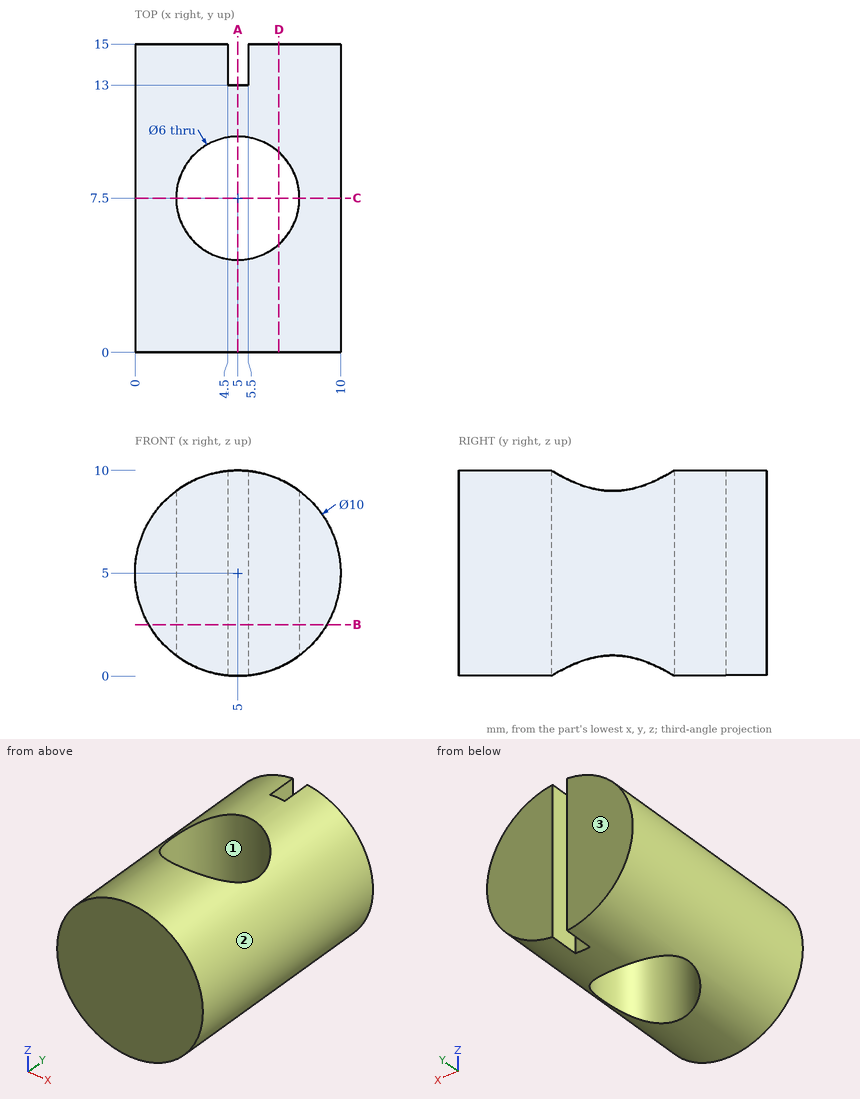
Could you check a few things on this drawing? It's one solid part, dimensions in mm from its lowest x, y, z. Coordinates: 2 decimals unless noted, no trailing zeros. Write each loop counter-clockwise with the first axis right and the second up, starting at its lowest first coordinate (ties: lowest second). Pieces come first, ordered by that corner, then holes. Notation, with made-up numbers: (2, 46) - (15, 46) arc R35 cw to (15, 78) - close; hole circle Ø11 at (87.5, 45). An arc over 180 degrees is marked (long way). Return JSON: item names as keys, results as strings. Group by question number.
Item 1: If we section it at A-A (x = 5): Write out the boundary of the cut face in (y, z).
Item 2: If we section it at B-B (z = 2.5): Write out the boundary of the cut face in (x, y), then the cut area to 3 significant figures.
Item 3: If we section it at C-C (y = 7.5): Write out the boundary of the cut face in (x, z).
Item 4: We'd pull the mould along X, two halves only. Please class the marked faces 1, 2 and 3: pulls with the +X half, pulls with the -X half, needs draft (parallel to the pull), parting line crosses it, or undercut.
Item 5: Please list where these lines run through material, in increasing order: probe 1 along Y at (x, z) = (5, 6.5); probe 2 along Y at (x, z) = (7, 4); probe 3 along Z at (x, y) = (1, 5.5).
Item 6: I'm going to push flat-ended pins straight in: pin 1 Ø3 at (y, z) = (3.5, 1.5) entering from -X; pin 2 Ø3 at (y, z) = (6, 8) entering from -X; pin 3 Ø0.5 at (x, z) = (5, 6.5) entering from +Y. Where does each tip first touch, or does it pass through?
Item 7: If we section it at D-D (x = 7): Write out the boundary of the cut face in (y, z), then the cut area to 3 significant figures.
Return value:
{
 "1": {"outline": "(0, 0) - (4.5, 0) - (4.5, 10) - (0, 10) - close; (10.5, 0) - (13, 0) - (13, 10) - (10.5, 10) - close"},
 "2": {"outline": "(0.67, 0) - (9.33, 0) - (9.33, 15) - (5.5, 15) - (5.5, 13) - (4.5, 13) - (4.5, 15) - (0.67, 15) - close; hole circle Ø6 at (5, 7.5)", "area": "99.6 mm^2"},
 "3": {"outline": "(2, 1) - (2, 9) arc R5 ccw to start; (8, 1) arc R5 ccw to (8, 9) - close"},
 "4": {"face 1": "undercut", "face 2": "parting line crosses it", "face 3": "needs draft"},
 "5": {"probe 1": "y = 0 to 4.5, 10.5 to 13", "probe 2": "y = 0 to 5.26, 9.74 to 15", "probe 3": "z = 2 to 8"},
 "6": {"pin 1": "stops at x = 0.42", "pin 2": "stops at x = 0.23", "pin 3": "stops at y = 13"},
 "7": {"outline": "(0, 0.42) - (5.26, 0.42) - (5.26, 9.58) - (0, 9.58) - close; (9.74, 0.42) - (15, 0.42) - (15, 9.58) - (9.74, 9.58) - close", "area": "96.5 mm^2"}
}
